from build123d import *

# Parameters (mm, degrees)
BOSS_EXTRUDE1_DEPTH = 160
BOSS_EXTRUDE2_START = 12
BOSS_EXTRUDE2_DEPTH = 12
BOSS_EXTRUDE3_START = -160
BOSS_EXTRUDE3_DEPTH = 12
SKETCH3_R           = 2.6
CUT_EXTRUDE1_DEPTH  = 12


with BuildPart() as part:
    # Sketch1 → Boss-Extrude1 (new body)
    with BuildSketch(Plane(origin=(0, 0, 0), x_dir=(1, 0, 0), z_dir=(0, 1, 0))):
        with BuildLine():
            Line((0, 2), (-6.1, 2))
            Line((-6.1, 2), (-6.1, 4))
            ThreePointArc((-6.1, 4), (-5.807106781, 4.707106781), (-5.1, 5))
            Line((-5.1, 5), (-1.05, 5))
            Line((-1.05, 5), (-1.05, 16))
            ThreePointArc((-1.05, 16), (-0.757106781, 16.707106781), (-0.05, 17))
            Line((-0.05, 17), (5.85, 17))
            ThreePointArc((5.85, 17), (6.557106781, 16.707106781), (6.85, 16))
            Line((6.85, 16), (6.85, 5))
            Line((6.85, 5), (10.9, 5))
            ThreePointArc((10.9, 5), (11.607106781, 4.707106781), (11.9, 4))
            Line((11.9, 4), (11.9, 2))
            Line((11.9, 2), (0, 2))
        make_face()
    extrude(amount=BOSS_EXTRUDE1_DEPTH)

    # Sketch2 → Boss-Extrude2 (add)
    with BuildSketch(Plane.XZ.offset(BOSS_EXTRUDE2_START)):
        with BuildLine():
            Line((11.9, -2), (-6.1, -2))
            Line((-6.1, -2), (-6.1, -4))
            ThreePointArc((-6.1, -4), (-5.807106781, -4.707106781), (-5.1, -5))
            Line((-5.1, -5), (10.9, -5))
            ThreePointArc((10.9, -5), (11.607106781, -4.707106781), (11.9, -4))
            Line((11.9, -4), (11.9, -2))
        make_face()
    extrude(amount=-BOSS_EXTRUDE2_DEPTH)

    # Sketch2<2> → Boss-Extrude3 (add)
    with BuildSketch(Plane.XZ.offset(BOSS_EXTRUDE3_START)):
        with BuildLine():
            Line((11.9, -2), (-6.1, -2))
            Line((-6.1, -2), (-6.1, -4))
            ThreePointArc((-6.1, -4), (-5.807106781, -4.707106781), (-5.1, -5))
            Line((-5.1, -5), (10.9, -5))
            ThreePointArc((10.9, -5), (11.607106781, -4.707106781), (11.9, -4))
            Line((11.9, -4), (11.9, -2))
        make_face()
    extrude(amount=-BOSS_EXTRUDE3_DEPTH)

    # Sketch3 → Cut-Extrude1 (cut)
    with BuildSketch(Plane(origin=(0, 0, -5), x_dir=(-1, 0, 0), z_dir=(0, 0, -1))):
        with Locations((-2.9, 166)):
            Circle(SKETCH3_R)
        with Locations((-2.9, -6)):
            Circle(SKETCH3_R)
    extrude(amount=-CUT_EXTRUDE1_DEPTH, mode=Mode.SUBTRACT)


solid = part.part
Check sheet for the modelled part. Datum: model origin and axes. Units: mm. A direction names the side the tool comes from. Round coordinates to 2 decimals unless told otherwise and drop trailing zeros. Loops run counter-clockwise (first coordinate to the right, second up) from the corner with the lowest first, then second, coordinate; pieces in that order, holes last. Notation, with made-up numbers: (77.5, -21) - (96.5, -21) arc R21 cw to (96.5, 18) - close; hole circle Ø9 at (61, 36). An arc over 180 degrees is marked (long way). Answer as CSV lines item,"result". Start each with the question number.
Item 1: Section check B-B (y = 166). Record the boundary of the cut face in (x, z), and give its area (3 significant figures).
Item 2: Depth check by flat-ended pin: P1, Ø5, axis at x = 3.5, z = -11, coming from the +Y side; P2, Ø1.5, axis at x = 1.5, z = -7, coming from the -Y side; P3, Ø5.5, axis at y = 110, z = -8.5, coming from the +X side. Enter the tip coordinate at first touch or a pass-through.
Item 3: Section check A-A (x = 2.9). Record the boundary of the cut face in (y, z).
Item 4: Set-up check for faces 5 (the flat face through (6.85, 79, -11)), 6 (the flat face through (3, 79, -17)), 7 (the flat face through (3, 160, -11)), 8 (the flat face through (3, 0, -11)): record each of +Z, -Z, +X, -X, +Y, -Y from which the full face is reachable in a straight line by a thin tool's end or side.
Item 5: Section check D-D (z = -12). Record the boundary of the cut face in (x, y).
Item 6: Scan lines: line 1 (Y direction, x = 2.9, z = -2.7); line 2 (X direction, y = 166, z = -3.5); line 3 (Y direction, x = 0.75, z = -15.5). Record each from-to range of solid material in increasing order. Write a range as [from, to].
Item 7: Release check for a two-part mould opening along X. For faces 1 (the flat face through (-1.05, 79, -10)), 2 (the flat face through (3, -12, -3)), 3 (the cylindrical face through (3.46, 163.46, -3.52)), 4 (the cylindrical face through (3.238, -3.422, -3.521)) record: +X half, -X half, draft (parallel to the pull), parting line (faces both ways), or undercut.
Item 8: Section check C-C (y = 48). Record the boundary of the cut face in (x, z).
Report:
1,outline,"(-6.1, -4) arc R1 ccw to (-5.1, -5) - (0.3, -5) - (0.3, -2) - (-6.1, -2) - close; (5.5, -5) - (10.9, -5) arc R1 ccw to (11.9, -4) - (11.9, -2) - (5.5, -2) - close"
1,area,"38.0 mm2"
2,P1,"stops at y = 160"
2,P2,"stops at y = 0"
2,P3,"stops at x = 6.85"
3,outline,"(-12, -5) - (-8.6, -5) - (-8.6, -2) - (-12, -2) - close; (-3.4, -5) - (0, -5) - (0, -17) - (160, -17) - (160, -5) - (163.4, -5) - (163.4, -2) - (-3.4, -2) - close; (168.6, -5) - (172, -5) - (172, -2) - (168.6, -2) - close"
4,face 5,"-Z, +X, +Y, -Y"
4,face 6,"-Z, +X, -X, +Y, -Y"
4,face 7,"-Z, +X, -X, +Y"
4,face 8,"-Z, +X, -X, -Y"
5,outline,"(-1.05, 0) - (6.85, 0) - (6.85, 160) - (-1.05, 160) - close"
6,line 1,"y = [-12, -8.6], [-3.4, 163.4], [168.6, 172]"
6,line 2,"x = [-6.1, 0.3], [5.5, 11.9]"
6,line 3,"y = [0, 160]"
7,face 1,"-X half"
7,face 2,"draft"
7,face 3,"undercut"
7,face 4,"undercut"
8,outline,"(-6.1, -4) arc R1 ccw to (-5.1, -5) - (-1.05, -5) - (-1.05, -16) arc R1 ccw to (-0.05, -17) - (5.85, -17) arc R1 ccw to (6.85, -16) - (6.85, -5) - (10.9, -5) arc R1 ccw to (11.9, -4) - (11.9, -2) - (-6.1, -2) - close"
